```python
from build123d import *

# Parameters (mm, degrees)
F1_DEPTH = 9.525


with BuildPart() as f1:
    # F0 (on Top) → F1 (new body)
    with BuildSketch(Plane.XY):
        with BuildLine():
            Line((0, 2.3), (-388.263155, 2.3))
            ThreePointArc((-388.263155, 2.3), (-401.840755, -11.2776), (-388.263155, -24.8552))
            Line((-388.263155, -24.8552), (-67.131578, -24.8552))
            ThreePointArc((-67.131578, -24.8552), (-64.457855, -25.139838), (-61.903982, -25.980994))
            Line((-61.903982, -25.980994), (-11.038081, -48.955043))
            ThreePointArc((-11.038081, -48.955043), (26.215066, -30.161652), (0, 2.3))
        make_face()
        with BuildLine():
            ThreePointArc((0, 0), (23.966614, -29.677434), (-10.091351, -46.858927))
            Line((-10.091351, -46.858927), (-60.957252, -23.884878))
            ThreePointArc((-60.957252, -23.884878), (-63.973638, -22.891387), (-67.131578, -22.5552))
            Line((-67.131578, -22.5552), (-388.263155, -22.5552))
            ThreePointArc((-388.263155, -22.5552), (-399.540755, -11.2776), (-388.263155, 0))
            Line((-388.263155, 0), (0, 0))
        make_face(mode=Mode.SUBTRACT)
    extrude(amount=F1_DEPTH)


solid = f1.part
```
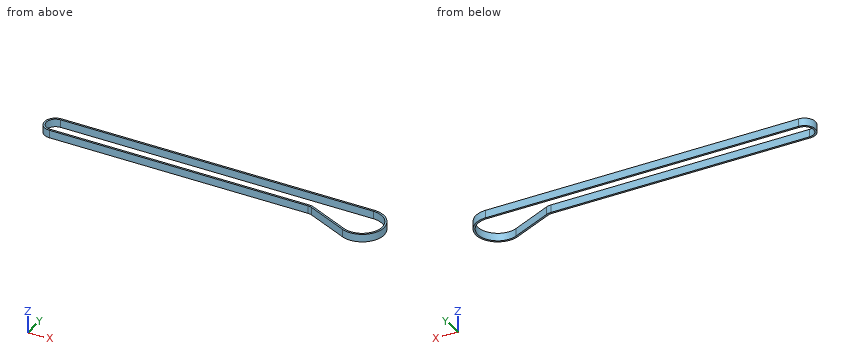
The model under review builds one solid part; all positions refer to its coordinate system, in mm. Round coordinates to 2 decimals unless told otherwise and drop trailing zeros. Order: outer loops, then holes, each group sorted by start corner. A loop starts at its lowest first (then second) coordinate and runs counter-clockwise, first axis right, second up. Notation, with made-up numbers: (65, 50) - (98, 50) arc R3 ccw to (98, 54) - close; hole circle Ø8 at (37.25, 24.5). An arc over 180 degrees is marked (long way). Answer in a Markdown table with one row per item.
(1) For line 1 (Y direction, x = 0, z = 4); line 2 (Y direction, x = -382.5, z = 8.75); line 3 (X direction, y = -46, z = 9), list the stretches that pass through material, from the lowest coordinate up. Write a range as from..to.
Result set:
| item | result |
|---|---|
| line 1 | y = -51.33..-49.03, 0..2.3 |
| line 2 | y = -24.86..-22.56, 0..2.3 |
| line 3 | x = -17.58..-11.99, 11.81..16.05 |
(2) Take a section at C-C on y = -15. Write out the cut boundary in (x, z) (3 decimals), plus the area to 3 significant figures.
Result set:
| item | result |
|---|---|
| outline | (-401.321, 0) - (-398.909, 0) - (-398.909, 9.525) - (-401.321, 9.525) - close; (22.594, 0) - (25.071, 0) - (25.071, 9.525) - (22.594, 9.525) - close |
| area | 46.6 mm2 |
(3) Clearance check with a flat-ended pin moving along its axis: P1, Ø3, axis at x = -250.5, z = 2.5, coming from the -Y side. State where the tip first meets the part, or that it passes through.
Result set:
| item | result |
|---|---|
| P1 | stops at y = -24.86 |
(4) Take a section at B-B on z = 3.25. Write out the cut boundary in (x, y), plus the area to 3 significant figures.
Result set:
| item | result |
|---|---|
| outline | (-388.26, -24.86) - (-67.13, -24.86) arc R12.7 cw to (-61.9, -25.98) - (-11.04, -48.96) arc R26.82 ccw (long way) to (0, 2.3) - (-388.26, 2.3) arc R13.58 ccw to start; hole (-388.26, -22.56) - (-67.13, -22.56) arc R15 cw to (-60.96, -23.88) - (-10.09, -46.86) arc R24.52 ccw (long way) to (0, 0) - (-388.26, 0) arc R11.28 ccw to start |
| area | 2,070 mm2 |
(5) Take a section at A-A on x = -136. Write out the cut boundary in (y, z) (3 decimals).
Result set:
| item | result |
|---|---|
| outline | (-24.855, 0) - (-22.555, 0) - (-22.555, 9.525) - (-24.855, 9.525) - close; (0, 0) - (2.3, 0) - (2.3, 9.525) - (0, 9.525) - close |
